Autodesk Inventor part; units mm, degrees
ref_plane "YZ Plane" through (0, 0, 0) normal (1, 0, 0) x (0, 1, 0)
ref_plane "XZ Plane" through (0, 0, 0) normal (0, 1, 0) x (-1, 0, 0)
ref_plane "XY Plane" through (0, 0, 0) normal (0, 0, 1) x (1, 0, 0)
sketch "Sketch1" plane through (0, 0, 0) normal (0, 0, 1) x (1, 0, 0)
  circle A0 centre (0, 0) radius 6.35
  dimension "d0" = 12.7
extrude "Extrusion1" add sketch "Sketch1" along normal blind 203.2
sketch "Sketch4" plane through (0, 0, 0) normal (0, 1, 0) x (-1, 0, 0)
  line L0 (0, 0) -> (0, 1.524)
  line L1 (6.35, 203.2) -> (-6.35, 203.2)
  line L2 (0, 203.2) -> (0, 201.676)
  circle A0 centre (0, 201.676) radius 1.27
  circle A1 centre (0, 1.524) radius 1.27
  dimension "d13" = 1.524
  dimension "d15" = 1.524
  dimension "d16" = 2.54
  dimension "d19" = 2.54
extrude "Extrusion4" cut sketch "Sketch4" along normal mid plane 15.24
sketch "Sketch8" plane through (0, 0, 0) normal (0, 1, 0) x (-1, 0, 0)
  line L0 (0, 0) -> (0, 50.8)
  circle A0 centre (0, 50.8) radius 1.27
  line L1 (0, 50.8) -> (0, 76.2)
  circle A1 centre (0, 76.2) radius 1.27
  line L2 (6.35, 203.2) -> (-6.35, 203.2)
  line L3 (0, 203.2) -> (0, 152.4)
  circle A2 centre (0, 152.4) radius 1.27
  line L4 (0, 152.4) -> (0, 127)
  circle A3 centre (0, 127) radius 1.27
  dimension "d50" = 50.8
  dimension "d51" = 2.54
  dimension "d58" = 25.4
  dimension "d59" = 2.54
  dimension "d60" = 50.8
  dimension "d61" = 2.54
  dimension "d62" = 25.4
  dimension "d63" = 2.54
extrude "Extrusion10" cut sketch "Sketch8" along normal mid plane 25.4
properties part number "Straw"
Input: part model. Units: mm. Frame: model coordinates. Coordinates: 2 decimals unless noted, no trailing zeros. Loops run counter-clockwise (first coordinate to the right, second up) from the corner with the lowest first, then second, coordinate; pieces in that order, holes last. Notation, with made-up numbers: M 12.5,50 L 55.5,50 A21 cw 55.5,57 Z; hole C 47.25,74 d5. An arc over 180 degrees is marked long. Use a Markdown table: item, result. Add a question column.
1) Draft query along X for faces 1 (the flat face through (0, 0, 203.2)), 2 (the cylindrical face through (-1.38, 6.2, 100.18)). Return one class per face: +X half, -X half, draft (parallel to the pull), parting line (faces both ways), or undercut.
2) Section B-B, the plane x = 3.75. Return the cut outline in (y, z), plus the area to 3 significant figures.
3) Pin query (flat end, axial travel): P1, Ø4, axis at x = -4.5, z = 60.5, coming from the -Y side; P2, Ø2, axis at y = -4, z = 96, coming from the -X side. Return the tip coordinate at first contact, or that it passes through.
4) Section A-A, the plane z = 115. Return the cut outline in (x, y).
5) Line query: L1, parallel to X at y = 1, z = 50.8; L2, parallel to X at y = 0.5, z = 43. Output: solid intervals per line, ascending. Write a range as from..to.
Answer below:
| question | item | result |
|---|---|---|
| 1 | face 1 | draft |
| 1 | face 2 | parting line |
| 2 | outline | M -5.12,0 L 5.12,0 L 5.12,203.2 L -5.12,203.2 Z |
| 2 | area | 2,080 mm2 |
| 3 | P1 | y = -5.84 |
| 3 | P2 | x = -5.6 |
| 4 | outline | C 0,0 d12.7 |
| 5 | L1 | -6.27..-1.27, 1.27..6.27 |
| 5 | L2 | -6.33..6.33 |
